from build123d import *

# Parameters (mm, degrees)
PAD_DEPTH       = 70
POCKET_DEPTH    = 3
SKETCH002_W     = 17.516219
SKETCH002_H     = 25.036772
POCKET001_DEPTH = 5
POCKET002_DEPTH = 4
SKETCH004_W     = 4.283857
SKETCH004_H     = 6.092597
POCKET003_DEPTH = 4
SKETCH005_W     = 5.455842
SKETCH005_H     = 7.092594
POCKET004_DEPTH = 4
POCKET005_DEPTH = 4


with BuildPart() as part:
    # Sketch → Pad (new body)
    with BuildSketch(Plane.XZ):
        Polygon((-30.042765, 9.957636), (30.084745, 9.957636), (30.084745, 49.997265), (0, 80.418144), (-30.042765, 50.004828), align=None)
    extrude(amount=PAD_DEPTH)

    # Sketch001 (on Face7 of Pad) → Pocket (cut)
    with BuildSketch(Plane.XZ.offset(70)):
        Polygon((-25.712206, 50.291458), (0, 76.657417), (26.325865, 50.291458), align=None)
    extrude(amount=-POCKET_DEPTH, mode=Mode.SUBTRACT)

    # Sketch002 (on Face5 of Pocket) → Pocket001 (cut)
    with BuildSketch(Plane.XZ.offset(70)):
        with Locations((-11.08819, 22.555024)):
            Rectangle(SKETCH002_W, SKETCH002_H)
    extrude(amount=-POCKET001_DEPTH, mode=Mode.SUBTRACT)

    # Sketch003 (on Face5 of Pocket001) → Pocket002 (cut)
    with BuildSketch(Plane.XZ.offset(70)):
        Polygon((12.177204, 35.510704), (11.921955, 41.636688), (17.665068, 41.636688), (17.665068, 35.255455), align=None)
    extrude(amount=-POCKET002_DEPTH, mode=Mode.SUBTRACT)

    # Sketch004 (on Face5 of Pocket002) → Pocket003 (cut)
    with BuildSketch(Plane.XZ.offset(70)):
        with Locations((22.218716, 38.549026)):
            Rectangle(SKETCH004_W, SKETCH004_H)
    extrude(amount=-POCKET003_DEPTH, mode=Mode.SUBTRACT)

    # Sketch005 (on Face5 of Pocket003) → Pocket004 (cut)
    with BuildSketch(Plane.XZ.offset(70)):
        with Locations((15.162952, 29.507296)):
            Rectangle(SKETCH005_W, SKETCH005_H)
    extrude(amount=-POCKET004_DEPTH, mode=Mode.SUBTRACT)

    # Sketch006 (on Face5 of Pocket004) → Pocket005 (cut)
    with BuildSketch(Plane.XZ.offset(70)):
        Polygon((20.12318, 32.68227), (20.12318, 25.923292), (25.454206, 26.113686), (25.454206, 32.68227), align=None)
    extrude(amount=-POCKET005_DEPTH, mode=Mode.SUBTRACT)


solid = part.part
Here's how the part is built. I have some questions about the finished solid (model axes, mm). A direction names the side the tool comes from. Round coordinates to 2 decimals unless told otherwise and drop trailing zeros. Loops run counter-clockwise (first coordinate to the right, second up) from the corner with the lowest first, then second, coordinate; pieces in that order, holes last.
1. If we section it at C-C on x = 10.5: Write out the boundary of the cut face in (y, z), plus the area to 3 significant figures.
Answer list:
outline: (-70, 9.96) - (0, 9.96) - (0, 69.8) - (-70, 69.8) - (-70, 66.14) - (-67, 66.14) - (-67, 50.29) - (-70, 50.29) - close
area: 4,140 mm2
2. If we section it at A-A on y = -41.5: Write out the boundary of the cut face in (x, z), plus the area to 3 significant figures.
Answer list:
outline: (-30.04, 9.96) - (30.08, 9.96) - (30.08, 50) - (0, 80.42) - (-30.04, 50) - close
area: 3,320 mm2
3. If we section it at B-B on z = 29.5: Write out the boundary of the cut face in (x, y), plus the area to 3 significant figures.
Answer list:
outline: (-30.04, -70) - (-19.85, -70) - (-19.85, -65) - (-2.33, -65) - (-2.33, -70) - (12.44, -70) - (12.44, -66) - (17.89, -66) - (17.89, -70) - (20.12, -70) - (20.12, -66) - (25.45, -66) - (25.45, -70) - (30.08, -70) - (30.08, 0) - (-30.04, 0) - close
area: 4,080 mm2
4. If I drill on line 1 along Y through (x, z) = (7.5, 69); line 2 along Y through (x, z) = (-8, 20); line 3 along Z through (x, y) = (-2.5, -37.5), over which ranges is the centre line in solid material (lowest first)?
Answer list:
line 1: y = -67 to 0
line 2: y = -65 to 0
line 3: z = 9.96 to 77.89
5. If we section it at D-D on z = 17: Write out the boundary of the cut face in (x, y).
Answer list:
outline: (-30.04, -70) - (-19.85, -70) - (-19.85, -65) - (-2.33, -65) - (-2.33, -70) - (30.08, -70) - (30.08, 0) - (-30.04, 0) - close
6. We'd pull the mould along X, two halves only. Please class faces 1 (the face through (-13.036, -68.521, 63.29)), 2 (the face through (-14.811, -34.51, 65.424)), 3 (the face through (0, 0, 38)): +X half, -X half, draft (parallel to the pull), parting line (faces both ways), or undercut.
Answer list:
face 1: undercut
face 2: -X half
face 3: draft
7. For P1, Ø6, axis at x = 15.5, z = 30, coming from the -Y side; P2, Ø1.5, axis at x = -4, y = -68, coming from the +Z side; P3, Ø3, axis at y = -28.5, z = 55, coming from the +X side; P4, Ø1.5, axis at x = 8.5, z = 67, coming from the -Y side, each with a flat end and sliding along its axis, tell me the tip position at first contact or that it passes through.
Answer list:
P1: stops at y = -70
P2: stops at z = 77.13
P3: stops at x = 26.62
P4: stops at y = -67
8. Which directions (+Z, -Z, +X, -X, +Y, -Y) give clear straight access to the entire face, cutting with the end or side of a thin tool? Please do faces 4 (the face through (-30.043, -35, 30)), 5 (the face through (23, -66, 29)).
Answer list:
face 4: +Z, -Z, -X, +Y, -Y
face 5: -Y
